Autodesk Inventor part; units mm, degrees
ref_plane "YZ Plane" through (0, 0, 0) normal (1, 0, 0) x (0, 1, 0)
ref_plane "XZ Plane" through (0, 0, 0) normal (0, 1, 0) x (-1, 0, 0)
ref_plane "XY Plane" through (0, 0, 0) normal (0, 0, 1) x (1, 0, 0)
sketch "Sketch1" plane through (0, 0, 0) normal (1, 0, 0) x (0, 1, 0)
  circle A0 centre (500, 0) radius 5
  circle A1 centre (-500, 0) radius 5
  arc A2 (500, -7.5) -> (500, 7.5) centre (500, 0) ccw
  arc A3 (-500, 7.5) -> (-500, -7.5) centre (-500, 0) ccw
  line L0 (500, -7.5) -> (-500, -7.5)
  line L1 (500, 7.5) -> (-500, 7.5)
  line L2 (-480, 5) -> (480, 5)
  line L3 (480, 5) -> (480, -5)
  line L4 (480, -5) -> (-480, -5)
  line L5 (-480, -5) -> (-480, 5)
  line L6 (-480, 5) -> (480, -5) construction
  line L7 (480, 5) -> (-480, -5) construction
  point P0 (0, 0)
  dimension "d0" = 10
  dimension "d1" = 10
  dimension "d2" = 15
  dimension "d3" = 15
  dimension "d4" = 1000
  dimension "d5" = 1000
  dimension "d6" = 960
  dimension "d7" = 10
extrude "Extrusion1" add sketch "Sketch1" along normal blind 1200
properties part number "Conveyer Belt"
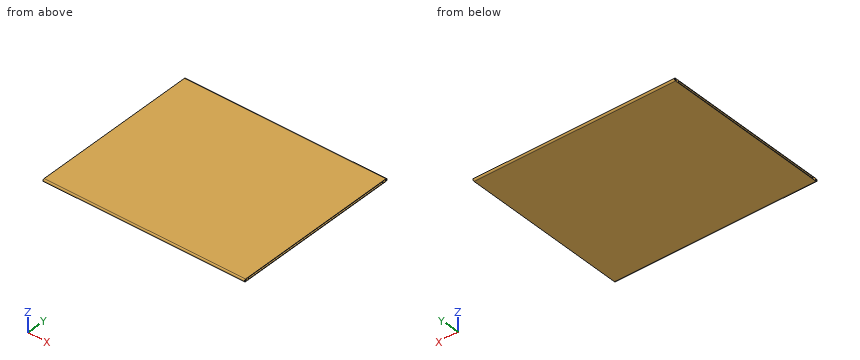
Design review of the part built by this model. Coordinates are the model's own, in mm. Round coordinates to 2 decimals unless told otherwise and drop trailing zeros. Write each loop counter-clockwise with the first axis right and the second up, starting at its lowest first coordinate (ties: lowest second). Pieces come first, ordered by that corner, then holes. Notation, with made-up numbers: (-34, 67) - (-21, 67) arc R19 cw to (-21, 92) - close; hole circle Ø6 at (26, 85.25). An arc over 180 degrees is marked (long way). Use a Markdown table: item, result. Add a question column.
1. Wall thickness on probe 1 along Y at (x, z) = (258, 0.5); probe 2 along Y at (x, z) = (523.5, 1.25); probe 3 along Z at (x, y) = (636, -349.5): over which ranges is each line inside the solid? List them lowest first.
2. We need section B-B (z = 0). State the section outline as (x, y) points.
3. We need section C-C (y = -245). State the section outline as (x, z) points.
4. Clearance check with flat-ended pins moving along their axes: pin 1 (5 mm diameter, centred on x = 692, z = -4.5, fed in from -Y); pin 2 (1.5 mm diameter, centred on y = 367.5, z = -4, fed in from -X). State where each tip first meets the part, or that it passes through.
5. We need section A-A (x = 904.5). State the section outline as (y, z) points, then the cut area to 3 significant figures.
Output:
| question | item | result |
|---|---|---|
| 1 | probe 1 | y = -507.48 to -504.97, -495.03 to -480, 480 to 495.03, 504.97 to 507.48 |
| 1 | probe 2 | y = -507.4 to -504.84, -495.16 to -480, 480 to 495.16, 504.84 to 507.4 |
| 1 | probe 3 | z = -7.5 to -5, 5 to 7.5 |
| 2 | outline | (0, -507.5) - (1200, -507.5) - (1200, -505) - (0, -505) - close; (0, -495) - (1200, -495) - (1200, -480) - (0, -480) - close; (0, 480) - (1200, 480) - (1200, 495) - (0, 495) - close; (0, 505) - (1200, 505) - (1200, 507.5) - (0, 507.5) - close |
| 3 | outline | (0, -7.5) - (1200, -7.5) - (1200, -5) - (0, -5) - close; (0, 5) - (1200, 5) - (1200, 7.5) - (0, 7.5) - close |
| 4 | pin 1 | stops at y = -507.23 |
| 4 | pin 2 | passes through |
| 5 | outline | (-500, -7.5) - (500, -7.5) arc R7.5 ccw to (500, 7.5) - (-500, 7.5) arc R7.5 ccw to start; hole circle Ø10 at (-500, 0); hole (-480, -5) - (480, -5) - (480, 5) - (-480, 5) - close; hole circle Ø10 at (500, 0) |
| 5 | area | 5,420 mm2 |
